Geometry check sheet. Reference: drawing and pictorial views, mm from the part's lowest x, y, z. Give positions to 0.01 mm unless a question says otherwise; leave off trailing zeros. Order: outer loops, then holes, each group sorted by start corner. A loop starts at its lowest first (then second) coordinate and runs counter-clockwise, first axis right, second up. Notation, with made-up numbers: (0.25, 10.25) -> (25.25, 10.25) arc R28 cw to (25.25, 29.25) -> close; hole circle Ø6 at (85.5, 66). An arc over 180 degrees is marked (long way). Write each question's results on one line, items separated by ' | '.
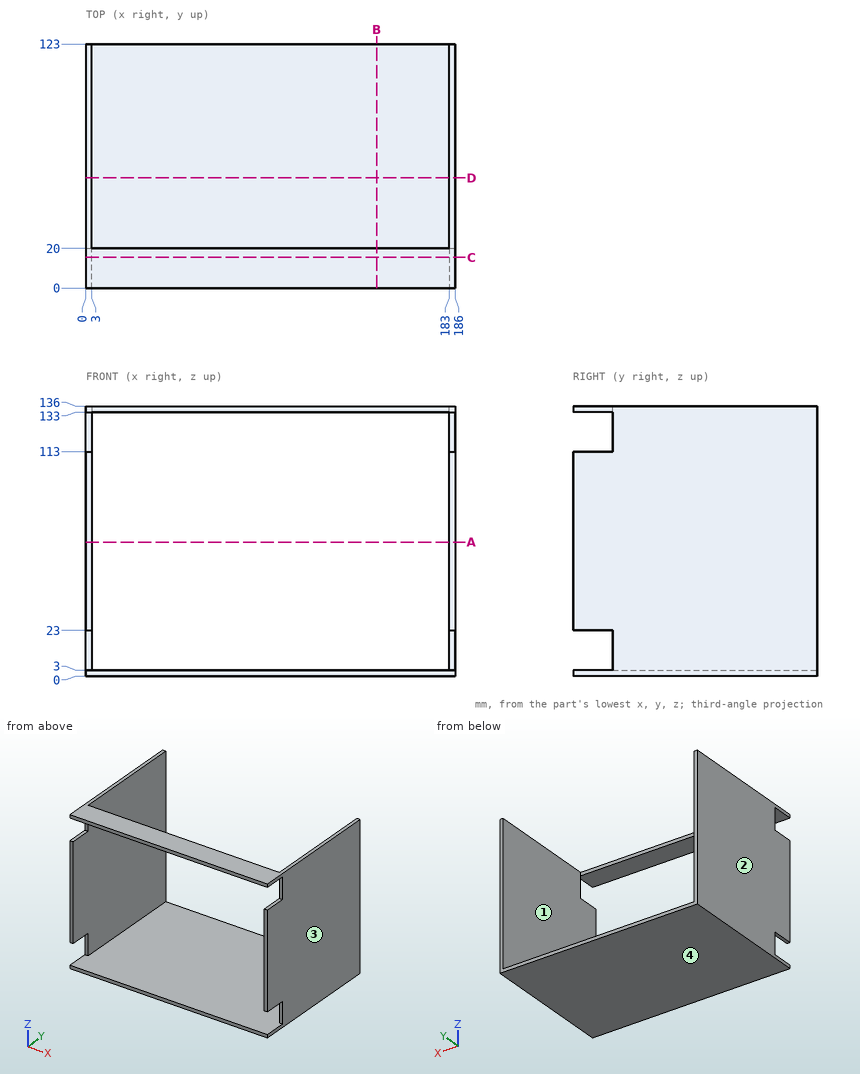
1. Section check A-A on z = 67.5. Record the cut outline in (x, y).
Verdict:
outline: (0, 0) -> (3, 0) -> (3, 123) -> (0, 123) -> close; (183, 0) -> (186, 0) -> (186, 123) -> (183, 123) -> close
2. Section check C-C on y = 15.5. Record the cut outline in (x, z), then the cut area to 3 significant figures.
Verdict:
outline: (0, 0) -> (186, 0) -> (186, 3) -> (0, 3) -> close; (0, 23) -> (3, 23) -> (3, 113) -> (0, 113) -> close; (0, 133) -> (186, 133) -> (186, 136) -> (0, 136) -> close; (183, 23) -> (186, 23) -> (186, 113) -> (183, 113) -> close | area: 1,660 mm^2
3. Section check D-D on y = 55.5. Record the cut outline in (x, z).
Verdict:
outline: (0, 0) -> (186, 0) -> (186, 136) -> (183, 136) -> (183, 3) -> (3, 3) -> (3, 136) -> (0, 136) -> close
4. Section check B-B on x = 146.5. Record the cut outline in (y, z), then the cut area to 3 significant figures.
Verdict:
outline: (0, 0) -> (123, 0) -> (123, 3) -> (0, 3) -> close; (0, 133) -> (20, 133) -> (20, 136) -> (0, 136) -> close | area: 429 mm^2
5. Mould release check, pull along X, two halves, no side actions. Record for the marked faces 1, 2, 3 and 4: +X half, -X half, draft (parallel to the pull), parting line (faces both ways), or undercut.
Verdict:
face 1: undercut | face 2: -X half | face 3: +X half | face 4: draft
6. Material ranges on probe 1 along X at (y, z) = (18, 69); probe 2 along Z at (x, y) = (97, 13.5); probe 3 along Z at (x, y) = (102.5, 60), recorded low to high. Write a range as from..to.
Verdict:
probe 1: x = 0..3, 183..186 | probe 2: z = 0..3, 133..136 | probe 3: z = 0..3
7. Gauge pin test, flat ends, axial feed: pin 1 Ø0.9 at (x, z) = (184.5, 16) entering from -Y; pin 2 Ø5 at (x, y) = (158, 103) entering from +Z; pin 3 Ø3.5 at (x, z) = (94, 135) entering from +Y. Record the tip position at first contact, or that the pin passes through.
Verdict:
pin 1: stops at y = 20 | pin 2: stops at z = 3 | pin 3: stops at y = 20
